Geometry: see drawing. Coordinates: mm, zero at the bounding-box minimum. A direction names the side the tool comes from. Give positions to 0.01 mm unless a question says otherwise; leave off trailing zeros. Write each loop counter-clockwise with the first axis right and the second up, starting at its lowest first coordinate (ties: lowest second). Pieces come first, ordered by that corner, then holes. Notation, with made-up numbers: M 11.25,73 L 53.25,73 A18 ccw 53.25,101 Z; hole C 65,-4.75 d8. An arc over 180 degrees is marked long. Answer as a JSON object with one key per item and string values. Group by question number.
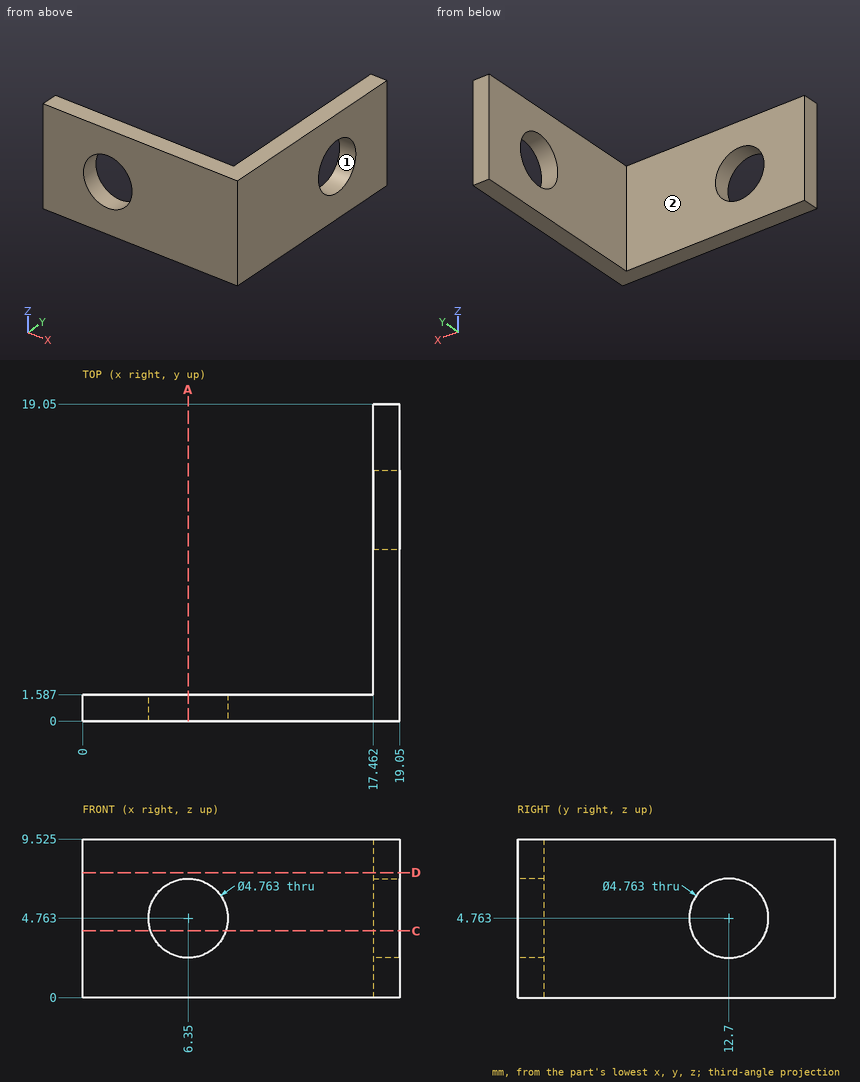
(1) Contact query for a flat-ended pin moving along its axis: pin 1 Ø5 at (x, z) = (3.5, 7.5) entering from +Y. Output: stop coordinate, or through.
(2) Section C-C, the plane z = 4. State how many separate pieces and enclosed holes the cut face has.
(3) Section A-A, the plane x = 6.35. Return loops of the section in (y, z) (1 decimal).
(4) Access query for the marked faces 1 and 2. Directions: +Z, -Z, +X, -X, +Y, -Y. A direction counts if a zero-diameter tool reaches every point of the face in a straight line with its end or side. Return the directions, or none.
(5) Section D-D, the plane z = 7.5. Return loops of the section in (x, y).
(6) Ray query, L1, parallel to Z at x = 6.35, y = 1.25 (1 decimal); L2, parallel to X at y = 8, z = 1; L3, parallel to Y at x = 5.25, z = 7.75. Return the intervals inside material, ascending. Write a range as [from, to].
Reported:
{
 "1": {"pin 1": "stops at y = 1.59"},
 "2": {"separate pieces": "3", "enclosed holes": "0"},
 "3": {"outline": "M 0,0 L 1.6,0 L 1.6,2.4 L 0,2.4 Z; M 0,7.1 L 1.6,7.1 L 1.6,9.5 L 0,9.5 Z"},
 "4": {"face 1": "+X, -X", "face 2": "+Z, -Z, -X, +Y"},
 "5": {"outline": "M 0,0 L 19.05,0 L 19.05,19.05 L 17.46,19.05 L 17.46,1.59 L 0,1.59 Z"},
 "6": {"L1": "z = [0, 2.4], [7.1, 9.5]", "L2": "x = [17.46, 19.05]", "L3": "y = [0, 1.59]"}
}
